Autodesk Inventor part; units mm, degrees
ref_plane "YZ Plane" through (0, 0, 0) normal (1, 0, 0) x (0, 1, 0)
ref_plane "XZ Plane" through (0, 0, 0) normal (0, 1, 0) x (-1, 0, 0)
ref_plane "XY Plane" through (0, 0, 0) normal (0, 0, 1) x (1, 0, 0)
sketch "Sketch1" plane through (0, 0, 0) normal (0, 0, 1) x (1, 0, 0)
  line L0 (0, 0) -> (81.43, 0)
  line L1 (81.43, 0) -> (81.43, 96.5)
  line L2 (81.43, 96.5) -> (0, 96.5)
  line L3 (0, 96.5) -> (0, 0)
  line L4 (5, 91.5) -> (76.43, 91.5)
  line L5 (76.43, 91.5) -> (76.43, 5)
  line L6 (76.43, 5) -> (5, 5)
  line L7 (5, 5) -> (5, 91.5)
  dimension "d1" = 81.43
  dimension "d2" = 96.5
  dimension "d3" = 5
  dimension "d4" = 5
  dimension "d5" = 5
  dimension "d6" = 5
extrude "Extrusion1" add sketch "Sketch1" against normal blind 3 contours L3 L2 L1 L0 | L4 L5 L6 L7
extrude "Extrusion2" add sketch "Sketch1" along normal blind 60
fillet "Fillet5" radius 2 2 edges at (0, 48.25, -3) (81.43, 48.25, -3)
fillet "Fillet6" radius 2 10 edges at (0.5858, 0, -2.4142) (0, 0, 29.5) (80.8442, 0, -2.4142) (81.43, 0, 29.5) (40.715, 0, -3) (80.8442, 96.5, -2.4142) (81.43, 96.5, 29.5) (0.5858, 96.5, -2.4142) (0, 96.5, 29.5) (40.715, 96.5, -3)
sketch "Sketch3" plane through (2, 0, 60) normal (0, -1, 0) x (1, 0, 0)
  line L0 (77.43, 0) -> (0, 0)
  line L1 (67.43, -39.1) -> (57.43, -39.1)
  line L2 (57.43, -39.1) -> (57.43, -31)
  line L3 (57.43, -31) -> (67.43, -31)
  line L4 (67.43, -31) -> (67.43, -39.1)
  line L5 (77.43, 0) -> (77.43, -61)
  line L6 (77.43, -61) -> (0, -61)
  line L7 (20, -31) -> (10, -31)
  line L8 (10, -31) -> (10, -39.1)
  line L9 (10, -39.1) -> (20, -39.1)
  line L10 (20, -39.1) -> (20, -31)
  line L11 (0, -61) -> (0, 0)
  point P0 (-2, -60)
  point P1 (77.43, -30)
  point P2 (76.43, -31)
  point P3 (1, -31)
  point P4 (0, -30)
  point P5 (10, -35.05)
  point P6 (73.8173, -31)
  point P7 (3.6124, -31)
  dimension "d38" = 10
  dimension "d39" = 8.1
  dimension "d40" = 10
  dimension "d41" = 21.9
  dimension "d42" = 10
  dimension "d43" = 8.1
  dimension "d44" = 21.9
  dimension "d45" = 10
extrude "Extrusion3" cut sketch "Sketch3" against normal blind 5 contours L1 L2 L3 L4 | L10 L9 L8 L7
sketch "Sketch4" plane through (2, 96.5, 60) normal (0, 1, 0) x (1, 0, 0)
  circle A0 centre (10, 35) radius 4
  line L0 (0, 61) -> (77.43, 61)
  line L1 (0, 0) -> (0, 61)
  circle A1 centre (67.43, 35) radius 4
  line L2 (77.43, 61) -> (77.43, 0)
  point P0 (-2, 60)
  point P1 (1, 31)
  point P2 (76.43, 31)
  point P3 (0, 30)
  point P4 (77.43, 30)
  point P5 (3.6123, 31)
  point P6 (73.8174, 31)
  dimension "d48" = 8
  dimension "d49" = 26
  dimension "d50" = 10
  dimension "d51" = 8
  dimension "d52" = 26
  dimension "d53" = 10
hole "Hole2" at (69.43, 96.5, 25) at (12, 96.5, 25) direction (0, -1, 0) diameter 2.95 depth 5 tip angle 118
equation "\"d52\" = d49"
properties part number "Component_shild_layered_TOPHAT"
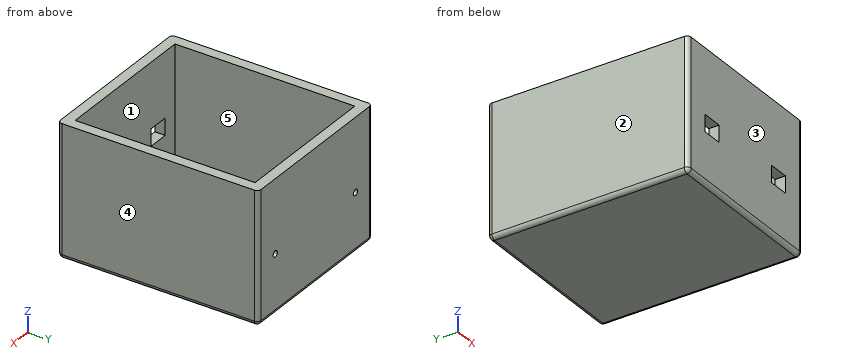
Work out the finished part from the listing and answer in its coordinate system (mm). Face numbers are marked on the shaded views. A direction names the side the tool comes from. Give positions to 0.01 mm unless a question says otherwise; leave off trailing zeros. Order: outer loops, then holes, each group sorted by start corner. A loop starts at its lowest first (then second) coordinate and runs counter-clockwise, first axis right, second up. Notation, with made-up numbers: (52, 49) -> (64, 49) arc R26 ccw to (64, 72) -> close; hole circle Ø2 at (-27.5, 84). An arc over 180 degrees is marked (long way). One line per item, written item: value.
Item 1: A tool of negligible diameter and unlimited length cuts with its end or side. For the marked faces 4 and 5, from which of +Z, -Z, +X, -X, +Y, -Y can it reach the whole face along a straight path? Write none if from no direction.
Answer sheet:
face 4: +Z, -Z, +X, +Y, -Y
face 5: +Z
Item 2: Flat-ended cylindrical pins translate along their axes: P1, Ø21.5, axis at x = 24, y = 50, coming from the +Z side; P2, Ø2.5, axis at x = 69.43, z = 25, coming from the +Y side. Find the tip coordinate at first contact, or state that the pin passes through.
Answer sheet:
P1: z = 0
P2: y = 5
Item 3: Find section C-C, the plane y = 79. Give the vertices of the cut face in (x, z), plus the area to 3 significant figures.
Answer sheet:
outline: (0, -1) arc R2 ccw to (2, -3) -> (79.43, -3) arc R2 ccw to (81.43, -1) -> (81.43, 60) -> (76.43, 60) -> (76.43, 0) -> (5, 0) -> (5, 60) -> (0, 60) -> close
area: 843 mm²
Item 4: Find section A-A, the plane x = 65. Give the vertices of the cut face in (y, z).
Answer sheet:
outline: (0, -1) arc R2 ccw to (2, -3) -> (94.5, -3) arc R2 ccw to (96.5, -1) -> (96.5, 60) -> (91.5, 60) -> (91.5, 0) -> (5, 0) -> (5, 20.9) -> (0, 20.9) -> close; (0, 29) -> (5, 29) -> (5, 60) -> (0, 60) -> close
Item 5: Find section D-D, the plane x = 24.5. Give the vertices of the cut face in (y, z).
Answer sheet:
outline: (0, -1) arc R2 ccw to (2, -3) -> (94.5, -3) arc R2 ccw to (96.5, -1) -> (96.5, 60) -> (91.5, 60) -> (91.5, 0) -> (5, 0) -> (5, 60) -> (0, 60) -> close
Item 6: Determine the mould class of the marked faces 1, 2 and 3 for opening direction X: released by +X, released by -X, zero draft, split by the parting line, or undercut.
Answer sheet:
face 1: undercut
face 2: released by -X
face 3: zero draft
Item 7: Straight lines are drawn through the part: probe 1 along X at (y, z) = (93, 25) (3 decimals); probe 2 along Y at (x, z) = (53, 57.5); probe 3 along X at (y, z) = (55, 22.5). For each, find the intervals that lie inside material, in ascending order.
Answer sheet:
probe 1: 0 to 10.525, 13.475 to 67.955, 70.905 to 81.43
probe 2: 0 to 5, 91.5 to 96.5
probe 3: 0 to 5, 76.43 to 81.43
Item 8: Find section B-B, the plane z = 25. Give the vertices of the cut face in (x, y) (3 decimals).
Answer sheet:
outline: (0, 2) arc R2 ccw to (2, 0) -> (12, 0) -> (12, 5) -> (5, 5) -> (5, 91.5) -> (10.525, 91.5) -> (10.525, 96.5) -> (2, 96.5) arc R2 ccw to (0, 94.5) -> close; (13.475, 91.5) -> (67.955, 91.5) -> (67.955, 96.5) -> (13.475, 96.5) -> close; (22, 0) -> (59.43, 0) -> (59.43, 5) -> (22, 5) -> close; (69.43, 0) -> (79.43, 0) arc R2 ccw to (81.43, 2) -> (81.43, 94.5) arc R2 ccw to (79.43, 96.5) -> (70.905, 96.5) -> (70.905, 91.5) -> (76.43, 91.5) -> (76.43, 5) -> (69.43, 5) -> close
